```python
from build123d import *

# Parameters (mm, degrees)
F0_W     = 65
F0_H     = 15
F1_DEPTH = 5
F2_R     = 10
F3_DEPTH = 40
F4_R     = 7.5
F5_DEPTH = 30


with BuildPart() as f1:
    # F0 (on Top) → F1 (new body)
    with BuildSketch(Plane.XY):
        Rectangle(F0_W, F0_H)
    extrude(amount=-F1_DEPTH)

    # F2 (on face) → F3 (join)
    with BuildSketch(Plane(origin=(0, 0, -5), x_dir=(1, 0, 0), z_dir=(0, 0, -1))):
        Circle(F2_R)
    extrude(amount=-F3_DEPTH)

    # F4 (on face) → F5 (join)
    with BuildSketch(Plane(origin=(0, 0, -5), x_dir=(1, 0, 0), z_dir=(0, 0, -1))):
        with BuildLine():
            ThreePointArc((-7.5, 0), (0, -7.5), (7.5, 0))
            ThreePointArc((7.5, 0), (0, 7.5), (-7.5, 0))
        make_face()
        with Locations((-22.5, 0)):
            Circle(F4_R)
        with BuildLine():
            ThreePointArc((30, 0), (22.5, 7.5), (15, 0))
            ThreePointArc((15, 0), (22.5, -7.5), (30, 0))
        make_face()
    extrude(amount=F5_DEPTH)


solid = f1.part
```
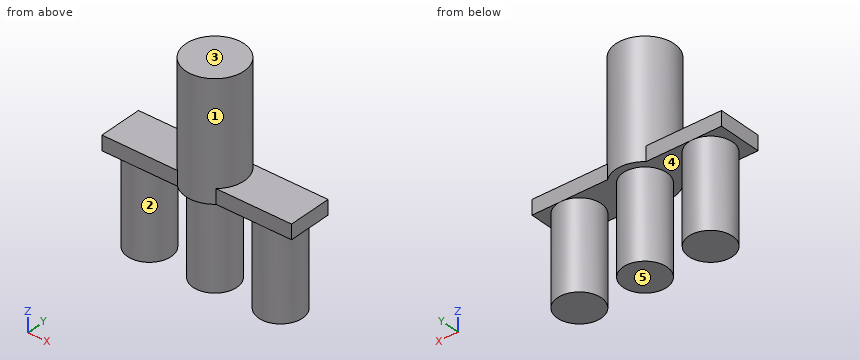
Could you check a few things on this model? Use its own coordinates, in mm. Face numbers are marked on the shaded views. A direction names the side the tool comes from. Coordinates: 2 decimals unless noted, no trailing zeros. Order: outer loops, then holes, each group sorted by start corner. A loop starts at its lowest first (then second) coordinate and runs counter-clockwise, first axis right, second up. Notation, with made-up numbers: M 38,-26 L 79,-26 A18 cw 79,-8 Z; hole C -27.5,21.5 d3. An arc over 180 degrees is marked long. Use a Markdown table: item, result. Add a question column.
Q1. If I drill on L1, parallel to X at y = -5.5, z = -29; L2, parallel to X at y = -0.5, z = -15.5; L3, parallel to Z at x = 14, y = 2.75, over which ranges is the centre line in solid material (lowest first)?
Q2. I want a section at B-B on z = -10. List the corners of the cut face in (x, y) for me, then the cut area to 3 significant figures.
Q3. I'm going to push flat-ended pins straight in: pin 1 (3 mm diameter, centred on x = -10, y = -1.5, fed in from -Z); pin 2 (12 mm diameter, centred on x = -19.5, y = -2, fed in from +Z); pin 3 (4 mm diameter, centred on x = -10.5, z = -18, fed in from +Y); pin 4 (5.5 mm diameter, centred on x = 24.5, z = -2.5, fed in from -Y). Where does each tip first touch, or does it pass through?
Q4. We'd pull the mould along X, two halves only. Please class the marked faces 1, 2 and 3: pulls with the +X half, pulls with the -X half, needs draft (parallel to the pull), parting line crosses it, or undercut.
Q5. I want a section at D-D on y = 3.75. List the corners of the cut face in (x, z) for me, then the cut area to 3 significant figures.
Q6. I want a section at C-C on x = 0. List the corners of the cut face in (y, z) for me.
Q7. I want a section at A-A on y = 0. List the corners of the cut face in (x, z) for me, then the cut area to 4 significant figures.
Q8. Which directions (+Z, -Z, +X, -X, +Y, -Y) give clear straight access to the entire face, cutting with the end or side of a thin tool? Please do the marked faces 4 and 5.
Checked values:
| question | item | result |
|---|---|---|
| 1 | L1 | -27.6 to -17.4, -5.1 to 5.1, 17.4 to 27.6 |
| 1 | L2 | -29.98 to -15.02, -7.48 to 7.48, 15.02 to 29.98 |
| 1 | L3 | -5 to 0 |
| 2 | outline | C -22.5,0 d15; C 0,0 d15; C 22.5,0 d15 |
| 2 | area | 530 mm² |
| 3 | pin 1 | z = -5 |
| 3 | pin 2 | z = 0 |
| 3 | pin 3 | through |
| 3 | pin 4 | y = -7.5 |
| 4 | face 1 | parting line crosses it |
| 4 | face 2 | undercut |
| 4 | face 3 | needs draft |
| 5 | outline | M -32.5,-5 L -29,-5 L -29,-35 L -16,-35 L -16,-5 L -6.5,-5 L -6.5,-35 L 6.5,-35 L 6.5,-5 L 16,-5 L 16,-35 L 29,-35 L 29,-5 L 32.5,-5 L 32.5,0 L 9.27,0 L 9.27,35 L -9.27,35 L -9.27,0 L -32.5,0 Z |
| 5 | area | 2,140 mm² |
| 6 | outline | M -10,-5 L -7.5,-5 L -7.5,-35 L 7.5,-35 L 7.5,-5 L 10,-5 L 10,35 L -10,35 Z |
| 7 | outline | M -32.5,-5 L -30,-5 L -30,-35 L -15,-35 L -15,-5 L -7.5,-5 L -7.5,-35 L 7.5,-35 L 7.5,-5 L 15,-5 L 15,-35 L 30,-35 L 30,-5 L 32.5,-5 L 32.5,0 L 10,0 L 10,35 L -10,35 L -10,0 L -32.5,0 Z |
| 7 | area | 2,375 mm² |
| 8 | face 4 | -Z |
| 8 | face 5 | -Z, +X, -X, +Y, -Y |
